from build123d import *

# Parameters (mm, degrees)
SKETCH_1_W          = 40
SKETCH_1_H          = 28
SKETCH_1_R          = 1.525
SKETCH_1_W_2        = 70
SKETCH_1_H_2        = 15
EXTRUDE_1_DEPTH     = 3
FILLET_1_R          = 4
SKETCH_2_W          = 54
SKETCH_2_H          = 48
CUT_EXTRUDE_1_DEPTH = 3
CHAMFER_1_SIZE      = 10
FILLET_2_R          = 4
FILLET_3_R          = 1


with BuildPart() as part:
    # 草图1 → 凸台-拉伸1 (new body)
    with BuildSketch(Plane.XY):
        Polygon((-35, 29), (-75, 14), (-35, 14), align=None)
        with Locations((-55, 0)):
            Rectangle(SKETCH_1_W, SKETCH_1_H)
        with Locations((-71, -10)):
            Circle(SKETCH_1_R, mode=Mode.SUBTRACT)
        with Locations((-71, 10)):
            Circle(SKETCH_1_R, mode=Mode.SUBTRACT)
        Polygon((-35, -14), (-75, -14), (-35, -29), align=None)
        with Locations((0, -21.5)):
            Rectangle(SKETCH_1_W_2, SKETCH_1_H_2)
        with Locations((-31, -25)):
            Circle(SKETCH_1_R, mode=Mode.SUBTRACT)
        with Locations((31, -25)):
            Circle(SKETCH_1_R, mode=Mode.SUBTRACT)
        Rectangle(SKETCH_1_W_2, SKETCH_1_H)
        with Locations((0, 21.5)):
            Rectangle(SKETCH_1_W_2, SKETCH_1_H_2)
        with Locations((-31, 25)):
            Circle(SKETCH_1_R, mode=Mode.SUBTRACT)
        with Locations((31, 25)):
            Circle(SKETCH_1_R, mode=Mode.SUBTRACT)
        Polygon((75, 14), (35, 29), (35, 14), align=None)
        with Locations((55, 0)):
            Rectangle(SKETCH_1_W, SKETCH_1_H)
        with Locations((71, -10)):
            Circle(SKETCH_1_R, mode=Mode.SUBTRACT)
        with Locations((71, 10)):
            Circle(SKETCH_1_R, mode=Mode.SUBTRACT)
        Polygon((75, -14), (35, -14), (35, -29), align=None)
    extrude(amount=EXTRUDE_1_DEPTH)

    # 圆角1
    fillet_1_edges = [part.edges().sort_by_distance(p)[0] for p in [
        (-35, 29, 1.5),
        (35, 29, 1.5),
        (75, 14, 1.5),
        (75, -14, 1.5),
        (35, -29, 1.5),
        (-35, -29, 1.5),
        (-75, -14, 1.5),
        (-75, 14, 1.5),
    ]]
    fillet(fillet_1_edges, radius=FILLET_1_R)

    # 草图2 → 切除-拉伸1 (cut)
    with BuildSketch(Plane.XY.offset(3)):
        Polygon((-56.436014311, 2.978767355), (-39.087503195, 22.127183961), (-64.985617819, 12.415390977), align=None)
        Polygon((-35, -20.681230304), (-35, 20.681230304), (-53.737243982, 0), align=None)
        Polygon((-39.087503195, -22.127183961), (-56.436014311, -2.978767355), (-64.985617819, -12.415390977), align=None)
        Polygon((-67, -8.681230304), (-59.134784639, 0), (-67, 8.681230304), align=None)
        Rectangle(SKETCH_2_W, SKETCH_2_H)
        Polygon((35, -20.681230304), (53.737243982, 0), (35, 20.681230304), align=None)
        Polygon((39.087503195, 22.127183961), (56.436014311, 2.978767355), (64.985617819, 12.415390977), align=None)
        Polygon((67, -8.681230304), (67, 8.681230304), (59.134784639, 0), align=None)
        Polygon((64.985617819, -12.415390977), (56.436014311, -2.978767355), (39.087503195, -22.127183961), align=None)
    extrude(amount=-CUT_EXTRUDE_1_DEPTH, mode=Mode.SUBTRACT)

    # 倒角1
    chamfer_1_edges = [part.edges().sort_by_distance(p)[0] for p in [
        (-27, -24, 1.5),
        (-27, 24, 1.5),
        (27, 24, 1.5),
        (27, -24, 1.5),
    ]]
    chamfer(chamfer_1_edges, length=CHAMFER_1_SIZE)

    # 圆角2
    fillet_2_edges = [part.edges().sort_by_distance(p)[0] for p in [
        (17, -24, 1.5),
        (-17, -24, 1.5),
        (-27, 14, 1.5),
        (-27, -14, 1.5),
        (27, 14, 1.5),
        (27, -14, 1.5),
        (-17, 24, 1.5),
        (17, 24, 1.5),
    ]]
    fillet(fillet_2_edges, radius=FILLET_2_R)

    # 圆角3
    fillet_3_edges = [part.edges().sort_by_distance(p)[0] for p in [
        (39.087503195, 22.127183961, 1.5),
        (64.985617819, 12.415390977, 1.5),
        (56.436014311, 2.978767355, 1.5),
        (35, -20.681230304, 1.5),
        (35, 20.681230304, 1.5),
        (53.737243982, 0, 1.5),
        (64.985617819, -12.415390977, 1.5),
        (39.087503195, -22.127183961, 1.5),
        (56.436014311, -2.978767355, 1.5),
        (67, 8.681230304, 1.5),
        (67, -8.681230304, 1.5),
        (59.134784639, 0, 1.5),
        (-56.436014311, -2.978767355, 1.5),
        (-39.087503195, -22.127183961, 1.5),
        (-64.985617819, -12.415390977, 1.5),
        (-53.737243982, 0, 1.5),
        (-35, 20.681230304, 1.5),
        (-35, -20.681230304, 1.5),
        (-67, 8.681230304, 1.5),
        (-59.134784639, 0, 1.5),
        (-67, -8.681230304, 1.5),
        (-64.985617819, 12.415390977, 1.5),
        (-39.087503195, 22.127183961, 1.5),
        (-56.436014311, 2.978767355, 1.5),
    ]]
    fillet(fillet_3_edges, radius=FILLET_3_R)


solid = part.part
Input: part model. Units: mm. Frame: model coordinates. Give positions to 0.01 mm unless a question says otherwise; leave off trailing zeros. Loops run counter-clockwise (first coordinate to the right, second up) from the corner with the lowest first, then second, coordinate; pieces in that order, holes last. Notation, with made-up numbers: (32, 12.25) - (80, 12.25) arc R13 cw to (80, 36.25) - close; hole circle Ø2 at (25, 77). An arc over 180 degrees is marked (long way). Use CSV: the item, a comma, the result in double quotes. Start each with the question number.
Item 1: Section A-A on x = 21.5. Return loops of the section in (y, z).
Item 2: Section C-C on y = 2. Return loops of the section in (x, z).
Item 3: Line query: line 1 (Y direction, x = -31, z = 0.7) (3 decimals); line 2 (Y direction, x = 56, z = 0.7) (3 decimals); line 3 (Y direction, x = -2, z = 1.5). Output: solid intervals per line, ascending.
Item 4: Mould query, pull axis X, two halves, no side actions, for faces 1 (the cylindrical face through (-74.27, 13.53, 1.52)), 2 (the flat face through (45.05, 9.59, 1.52)). Classes: pulls with the +X half, pulls with the -X half, needs draft (parallel to the pull), parting line crosses it, or undercut.
Item 5: Section B-B on x = -31. Return loops of the section in (y, z) (3 decimals), then the cut area to 3 significant figures.
Item 6: Section D-D on z = 2.45. State how many separate pieces and enclosed holes the cut face has, then the cut area to 3 significant figures.
Ans:
1,outline,"(-29, 0) - (-19.5, 0) - (-19.5, 3) - (-29, 3) - close; (19.5, 0) - (29, 0) - (29, 3) - (19.5, 3) - close"
2,outline,"(-75, 0) - (-67, 0) - (-67, 3) - (-75, 3) - close; (-60.95, 0) - (-51.93, 0) - (-51.93, 3) - (-60.95, 3) - close; (-35, 0) - (-27, 0) - (-27, 3) - (-35, 3) - close; (27, 0) - (35, 0) - (35, 3) - (27, 3) - close; (51.93, 0) - (60.95, 0) - (60.95, 3) - (51.93, 3) - close; (67, 0) - (75, 0) - (75, 3) - (67, 3) - close"
3,line 1,"y = -29 to -26.525, -23.475 to 23.475, 26.525 to 29"
3,line 2,"y = -21.125 to -15.785, -3.568 to 3.568, 15.785 to 21.125"
3,line 3,"y = -29 to -24, 24 to 29"
4,face 1,"pulls with the -X half"
4,face 2,"undercut"
5,outline,"(-29, 0) - (-26.525, 0) - (-26.525, 3) - (-29, 3) - close; (-23.475, 0) - (23.475, 0) - (23.475, 3) - (-23.475, 3) - close; (26.525, 0) - (29, 0) - (29, 3) - (26.525, 3) - close"
5,area,"156 mm2"
6,separate pieces,"1"
6,enclosed holes,"17"
6,area,"3,510 mm2"
